CAD build for the part. Positions are in the model's coordinates, mm. Face numbers are marked on the shaded views. A direction names the side the tool comes from. Coordinates: 2 decimals unless noted, no trailing zeros. Order: outer loops, then holes, each group sorted by start corner. A loop starts at its lowest first (then second) coordinate and runs counter-clockwise, first axis right, second up. Notation, with made-up numbers: (56.5, 5.25) - (95.5, 5.25) arc R30 cw to (95.5, 30.25) - close; hole circle Ø6 at (10, 36.25). An arc over 180 degrees is marked (long way). Return JSON: item names as keys, results as strings.
from build123d import *

# Parameters (mm, degrees)
SKETCH1_W           = 76.2
SKETCH1_H           = 63.5
BOSS_EXTRUDE1_DEPTH = 3.175
SKETCH3_W           = 12.7
SKETCH3_H           = 25.4
SKETCH3_R           = 1.5875
BOSS_EXTRUDE2_DEPTH = 3.175
FILLET1_R           = 2.54


with BuildPart() as part:
    # Sketch1 → Boss-Extrude1 (new body)
    with BuildSketch(Plane(origin=(0, 0, 0), x_dir=(1, 0, 0), z_dir=(0, 1, 0))):
        Rectangle(SKETCH1_W, SKETCH1_H)
    extrude(amount=-BOSS_EXTRUDE1_DEPTH)

    # Sketch3 → Boss-Extrude2 (add)
    with BuildSketch(Plane.XY.offset(31.75)):
        with Locations((-31.75, -15.875)):
            Rectangle(SKETCH3_W, SKETCH3_H)
        with Locations((-31.75, -26.19375)):
            Circle(SKETCH3_R, mode=Mode.SUBTRACT)
        with Locations((-31.75, -8.73125)):
            Circle(SKETCH3_R, mode=Mode.SUBTRACT)
    boss_extrude2 = extrude(amount=-BOSS_EXTRUDE2_DEPTH)

    # Mirror1: Boss-Extrude2 across plane
    add(boss_extrude2.mirror(Plane.XY))

    # Fillet1
    fillet1_edges = [part.edges().sort_by_distance(p)[0] for p in [
        (-38.1, -28.575, 30.1625),
        (-25.4, -3.175, 30.1625),
        (-25.4, -28.575, 30.1625),
        (-38.1, -28.575, -30.1625),
        (-25.4, -28.575, -30.1625),
        (-25.4, -3.175, -30.1625),
    ]]
    fillet(fillet1_edges, radius=FILLET1_R)


solid = part.part
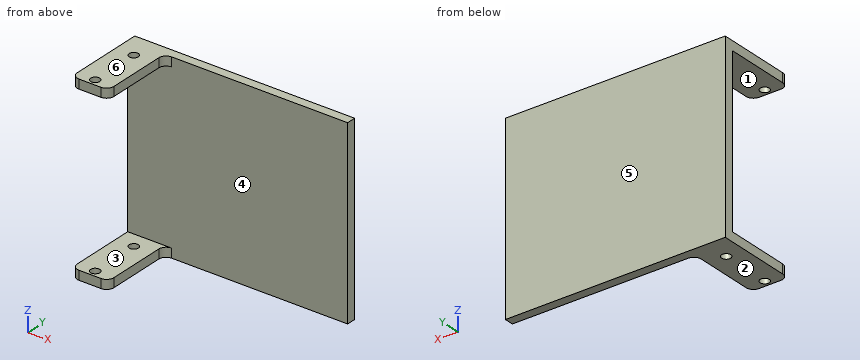
Item 1: Band-saw the part on B-B, the plane y = -17.5. List the corners of the cut face in (x, z) (3 decimals).
Findings below:
{"outline": "(-38.1, -31.75) - (-25.4, -31.75) - (-25.4, -28.575) - (-38.1, -28.575) - close; (-38.1, 28.575) - (-25.4, 28.575) - (-25.4, 31.75) - (-38.1, 31.75) - close"}
Item 2: Mould opens along Z. For the marked faces 3, 4, 5 and 6 say: released by +Z, released by -Z, zero draft, split by the parting line, or undercut.
Findings below:
{"face 3": "undercut", "face 4": "undercut", "face 5": "zero draft", "face 6": "released by +Z"}
Item 3: Which spindle directions (+Z, -Z, +X, -X, +Y, -Y) get a long thin tool onto all of the face, cutting with end or side? Do the marked faces 1 and 2. Say none if no direction does.
Findings below:
{"face 1": "+X, -X, -Y", "face 2": "-Z, +X, -X, +Y, -Y"}
Item 4: Band-saw the part on C-C, the plane z = 16. List the corners of the cut face in (x, y) (3 decimals).
Findings below:
{"outline": "(-38.1, -3.175) - (38.1, -3.175) - (38.1, 0) - (-38.1, 0) - close"}
Item 5: Band-saw the part on D-D, the plane x = 1.5. List the corners of the cut face in (y, z) (3 decimals).
Findings below:
{"outline": "(-3.175, -31.75) - (0, -31.75) - (0, 31.75) - (-3.175, 31.75) - close"}
Item 6: Band-saw the part on A-A, the plane x = -31.75. List the corners of the cut face in (y, z) (3 decimals).
Findings below:
{"outline": "(-28.575, -31.75) - (-27.781, -31.75) - (-27.781, -28.575) - (-28.575, -28.575) - close; (-28.575, 28.575) - (-27.781, 28.575) - (-27.781, 31.75) - (-28.575, 31.75) - close; (-24.606, -31.75) - (-10.319, -31.75) - (-10.319, -28.575) - (-24.606, -28.575) - close; (-24.606, 28.575) - (-10.319, 28.575) - (-10.319, 31.75) - (-24.606, 31.75) - close; (-7.144, -31.75) - (0, -31.75) - (0, 31.75) - (-7.144, 31.75) - (-7.144, 28.575) - (-3.175, 28.575) - (-3.175, -28.575) - (-7.144, -28.575) - close"}
Item 7: Drop flat-ended pins along their axis: P1, Ø10, axis at y = -13.5, z = 23, coming from the +X side; P2, Ø12, axis at x = -1, z = 19, coming from the -Y side (3 decimals); P3, Ø1.6, axis at y = -16.5, z = 29.5, coming from the +X side. Give the stop position or say it passes through.
Findings below:
{"P1": "passes through", "P2": "stops at y = -3.175", "P3": "stops at x = -25.4"}
Item 8: Wall check: L1, parallel to Y at x = -31.75, z = -29.7 (3 decimals); L2, parallel to Z at x = -33, y = -23.25 (3 decimals); L3, parallel to Y at x = -31, z = -29 (3 decimals). Give the ranges that are in metal, low to high. Write a range as [from, to].
Findings below:
{"L1": "y = [-28.575, -27.781], [-24.606, -10.319], [-7.144, 0]", "L2": "z = [-31.75, -28.575], [28.575, 31.75]", "L3": "y = [-28.575, -27.593], [-24.795, -10.13], [-7.332, 0]"}
